Model file for the job. Use its own axes, mm. A direction names the side the tool comes from. Round coordinates to 2 decimals unless told otherwise and drop trailing zeros. Loops run counter-clockwise (first coordinate to the right, second up) from the corner with the lowest first, then second, coordinate; pieces in that order, holes last. Notation, with made-up numbers: (33.5, -13) -> (56.5, -13) arc R28 ccw to (56.5, 7) -> close; hole circle Ø5 at (-33.75, -31.75). An arc over 180 degrees is marked (long way). Use a Markdown table: item, result.
from build123d import *

# Parameters (mm, degrees)
SKETCH_1_R          = 27.5
EXTRUDE_1_DEPTH     = 4
SKETCH_2_R          = 25.4
EXTRUDE_2_DEPTH     = 3.175
SKETCH_3_R          = 1.6
CUT_EXTRUDE_1_DEPTH = 40.547194907


with BuildPart() as part:
    # ｽｹｯﾁ1 → ﾎﾞｽ - 押し出し1 (new body)
    with BuildSketch(Plane.XY):
        Circle(SKETCH_1_R)
    extrude(amount=EXTRUDE_1_DEPTH)

    # ｽｹｯﾁ2 → ﾎﾞｽ - 押し出し2 (add)
    with BuildSketch(Plane(origin=(0, 0, 0), x_dir=(-1, 0, 0), z_dir=(0, 0, -1))):
        Circle(SKETCH_2_R)
    extrude(amount=EXTRUDE_2_DEPTH)

    # ｽｹｯﾁ3 → ｶｯﾄ - 押し出し1 (cut, through all)
    with BuildSketch(Plane(origin=(0, 0, -3.175), x_dir=(-1, 0, 0), z_dir=(0, 0, -1))):
        with Locations((0, 22.5)):
            Circle(SKETCH_3_R)
        with Locations((22.5, 0)):
            Circle(SKETCH_3_R)
        with Locations((0, -22.5)):
            Circle(SKETCH_3_R)
        with Locations((-22.5, 0)):
            Circle(SKETCH_3_R)
    extrude(amount=-CUT_EXTRUDE_1_DEPTH, mode=Mode.SUBTRACT)


solid = part.part
Q1. Band-saw the part on A-A, the plane x = 0. Give the cut face in (y, z) (3 decimals), plus the area to 3 significant figures.
Results list:
| item | result |
|---|---|
| outline | (-27.5, 0) -> (-25.4, 0) -> (-25.4, -3.175) -> (-24.1, -3.175) -> (-24.1, 4) -> (-27.5, 4) -> close; (-20.9, -3.175) -> (20.9, -3.175) -> (20.9, 4) -> (-20.9, 4) -> close; (24.1, -3.175) -> (25.4, -3.175) -> (25.4, 0) -> (27.5, 0) -> (27.5, 4) -> (24.1, 4) -> close |
| area | 335 mm² |
Q2. Band-saw the part on D-D, the plane x = 22.5. Give the cut face in (y, z) (3 decimals).
Results list:
| item | result |
|---|---|
| outline | (-15.811, 0) -> (-11.786, 0) -> (-11.786, -3.175) -> (-1.6, -3.175) -> (-1.6, 4) -> (-15.811, 4) -> close; (1.6, -3.175) -> (11.786, -3.175) -> (11.786, 0) -> (15.811, 0) -> (15.811, 4) -> (1.6, 4) -> close |
Q3. Band-saw the part on C-C, the plane z = 1.25. Give the cut face in (x, y), plus the area to 3 significant figures.
Results list:
| item | result |
|---|---|
| outline | circle Ø55 at (0, 0); hole circle Ø3.2 at (-22.5, 0); hole circle Ø3.2 at (0, -22.5); hole circle Ø3.2 at (0, 22.5); hole circle Ø3.2 at (22.5, 0) |
| area | 2,340 mm² |
Q4. Pull direction X, two halves, no side cores. Call faces 1 (the face through (20.974, 0.481, 0.362)), 2 (the face through (-5.961, -26.846, 1.972)), 3 (the face through (0, 0, -3.175)): released by +X, released by -X, zero draft, split by the parting line, or undercut.
Results list:
| item | result |
|---|---|
| face 1 | undercut |
| face 2 | split by the parting line |
| face 3 | zero draft |
Q5. Tool access for faces 4 (the face through (0.208, 24.086, 0.362)), 5 (the face through (5.506, -24.796, -1.565)): list every direction of +Z, -Z, +X, -X, +Y, -Y with a clear straight run to the whole face (end or side of a thin tool).
Results list:
| item | result |
|---|---|
| face 4 | +Z, -Z |
| face 5 | -Z |
Q6. Flat gauge pins, fed straight in: pin 1 (4 mm diameter, centred on y = 7, z = 3, fed in from +X); pin 2 (1 mm diameter, centred on x = 16, z = 3, fed in from +Y); pin 3 (2.5 mm diameter, centred on x = -22.5, y = 0, fed in from +Z). Where does each tip first touch, or does it go through?
Results list:
| item | result |
|---|---|
| pin 1 | stops at x = 27.04 |
| pin 2 | stops at y = 22.72 |
| pin 3 | passes through |
Q7. Drill centre lines: L1, parallel to Y at x = 0, z = 2.5; L2, parallel to Y at x = 23, z = 0.5; L3, parallel to Y at x = 22.5, z = 1. Where is each one in solid material? Low to high. Write a range as from..to.
Results list:
| item | result |
|---|---|
| L1 | y = -27.5..-24.1, -20.9..20.9, 24.1..27.5 |
| L2 | y = -15.07..-1.52, 1.52..15.07 |
| L3 | y = -15.81..-1.6, 1.6..15.81 |
